Work out the finished part from the listing and answer in its coordinate system (mm). Face numbers are marked on the shaded views. A direction names the side the tool comes from. Coordinates: 2 decimals unless noted, no trailing zeros. Order: outer loops, then holes, each group sorted by start corner. A loop starts at its lowest first (then second) coordinate and runs counter-clockwise, first axis right, second up.
1. The part is cut by section D-D, the plane x = -12.5. Give the vertices of the cut face in (y, z).
2. The part is cut by section B-B, the plane x = -2.5. Give the vertices of the cut face in (y, z), then the cut area to 3 significant figures.
3. Flat-ended cylindrical pins translate along their axes: pin 1 Ø1 at (y, z) = (18.5, 0) entering from +X; pin 2 Ø12 at (x, z) = (10, -8.5) entering from +Y; pin 3 Ø10 at (y, z) = (22, 4) entering from -X. Find the tip coordinate at first contact, or state that the pin passes through.
4. The part is cut by section A-A, the plane z = 0. Give the vertices of the cut face in (x, y).
5. The part is cut by section C-C, the plane y = 25. Give the vertices of the cut face in (x, z), then the cut area to 3 significant figures.
6. Find the intervals of material crossed by probe 1 along X at (y, z) = (1, 0); probe 2 along Z at (x, y) = (12.5, 1.9); probe 3 along Y at (x, z) = (17.5, 7), in increasing order.
7. A tool of negligible diameter and unlimited length cuts with its end or side. For the marked faces 1, 2 and 3, from which of +Z, -Z, +X, -X, +Y, -Y can it reach the whole face along a straight path? Write none if from no direction.
```python
from build123d import *

# Parameters (mm, degrees)
SKETCH1_W                  = 40
SKETCH1_H                  = 40
BOSS_EXTRUDE1_DEPTH        = 5
SKETCH4_W                  = 10
SKETCH4_H                  = 40
BOSS_EXTRUDE3_DEPTH        = 30
SKETCH5_R                  = 3
CUT_EXTRUDE4_DEPTH         = 26
FILLET1_R                  = 15
FILETE1_R                  = 10
ESBO_O1_R                  = 2.65
CORTE_EXTRUS_O1_DEPTH      = 31
CORTE_EXTRUS_O1_DEPTH_BACK = 6
ESBO_O2_R                  = 5
CORTE_EXTRUS_O2_DEPTH      = 31


with BuildPart() as part:
    # Sketch1 → Boss-Extrude1 (new body)
    with BuildSketch(Plane(origin=(0, 0, 0), x_dir=(1, 0, 0), z_dir=(0, 1, 0))):
        Rectangle(SKETCH1_W, SKETCH1_H)
    extrude(amount=BOSS_EXTRUDE1_DEPTH)

    # Sketch4 → Boss-Extrude3 (add)
    with BuildSketch(Plane(origin=(0, 5, 0), x_dir=(1, 0, 0), z_dir=(0, 1, 0))):
        Rectangle(SKETCH4_W, SKETCH4_H)
    extrude(amount=BOSS_EXTRUDE3_DEPTH)

    # Sketch5 → Cut-Extrude4 (cut, through all)
    with BuildSketch(Plane(origin=(5, 0, 0), x_dir=(0, 0, -1), z_dir=(1, 0, 0))):
        with Locations((0, 25)):
            Circle(SKETCH5_R)
    extrude(amount=-CUT_EXTRUDE4_DEPTH, mode=Mode.SUBTRACT)

    # Fillet1
    fillet1_edges = [part.edges().sort_by_distance(p)[0] for p in [
        (0, 35, -20),
        (0, 35, 20),
    ]]
    fillet(fillet1_edges, radius=FILLET1_R)

    # Filete1
    filete1_edges = [part.edges().sort_by_distance(p)[0] for p in [
        (5, 5, 0),
        (-5, 5, 0),
    ]]
    fillet(filete1_edges, radius=FILETE1_R)

    # Esboço1 → Corte-extrusão1 (cut, two sides)
    with BuildSketch(Plane(origin=(0, 5, 0), x_dir=(1, 0, 0), z_dir=(0, 1, 0))) as corte_extrus_o1_sk:
        with Locations((-12.5, 0)):
            Circle(ESBO_O1_R)
        with Locations((12.5, 0)):
            Circle(ESBO_O1_R)
    extrude(amount=CORTE_EXTRUS_O1_DEPTH, mode=Mode.SUBTRACT)
    extrude(corte_extrus_o1_sk.sketch, amount=-CORTE_EXTRUS_O1_DEPTH_BACK, mode=Mode.SUBTRACT)

    # Esboço2 → Corte-extrusão2 (cut, through all)
    with BuildSketch(Plane(origin=(0, 5, 0), x_dir=(1, 0, 0), z_dir=(0, 1, 0))):
        with Locations((-12.5, 0)):
            Circle(ESBO_O2_R)
        with Locations((12.5, 0)):
            Circle(ESBO_O2_R)
    extrude(amount=CORTE_EXTRUS_O2_DEPTH, mode=Mode.SUBTRACT)


solid = part.part
```
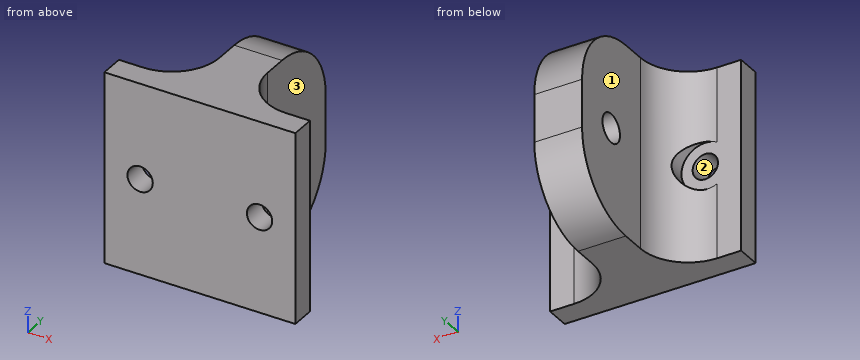
Geometry says:
1. outline: (0, -20) - (5.32, -20) - (5.32, -5) - (5, -5) - (5, -2.65) - (0, -2.65) - close; (0, 2.65) - (5, 2.65) - (5, 5) - (5.32, 5) - (5.32, 20) - (0, 20) - close
2. outline: (0, -20) - (20, -20) arc R15 ccw to (35, -5) - (35, 5) arc R15 ccw to (20, 20) - (0, 20) - close; hole circle Ø6 at (25, 0)
2. area: 1,280 mm2
3. pin 1: stops at x = 5
3. pin 2: stops at y = 35
3. pin 3: stops at x = -5
4. outline: (-20, 0) - (-15.15, 0) - (-15.15, 5) - (-20, 5) - close; (-9.85, 0) - (9.85, 0) - (9.85, 5) - (7.5, 5) - (7.5, 8.39) arc R10 cw to (5, 15) - (5, 22) - (-5, 22) - (-5, 15) arc R10 cw to (-7.5, 8.39) - (-7.5, 5) - (-9.85, 5) - close; (-5, 28) - (5, 28) - (5, 35) - (-5, 35) - close; (15.15, 0) - (20, 0) - (20, 5) - (15.15, 5) - close
5. outline: (-5, -19.14) - (5, -19.14) - (5, -3) - (-5, -3) - close; (-5, 3) - (5, 3) - (5, 19.14) - (-5, 19.14) - close
5. area: 323 mm2
6. probe 1: x = -20 to -15.15, -9.85 to 9.85, 15.15 to 20
6. probe 2: z = -20 to -2.65, 2.65 to 20
6. probe 3: y = 0 to 5
7. face 1: +Z, -Z, -X, +Y
7. face 2: +Y, -Y
7. face 3: +Z, -Z, +X, +Y
